from build123d import *

# Parameters (mm, degrees)
F0_W     = 63.5
F0_H     = 82.55
F1_DEPTH = 22.225
F2_R     = 2.38125
F3_DEPTH = 12.7
F4_R     = 2.38125
F5_DEPTH = 63.501
F6_R     = 1.27
F7_DEPTH = 25.4
F8_R     = 3.96875
F9_DEPTH = 3.81


with BuildPart() as f1:
    # F0 (on Front) → F1 (new body, symmetric)
    with BuildSketch(Plane.XZ):
        Rectangle(F0_W, F0_H)
    extrude(amount=F1_DEPTH, both=True)

    # F2 (on face) → F3 (cut)
    with BuildSketch(Plane.XY.offset(41.275)):
        Circle(F2_R)
    extrude(amount=-F3_DEPTH, mode=Mode.SUBTRACT)

    # F4 (on face) → F5 (cut, through all)
    with BuildSketch(Plane(origin=(-31.75, 0, 0), x_dir=(0, -1, 0), z_dir=(-1, 0, 0))):
        with Locations((0, 26.035)):
            Circle(F4_R)
        with Locations((0, -26.035)):
            Circle(F4_R)
    extrude(amount=-F5_DEPTH, mode=Mode.SUBTRACT)

    # F6 (on face) → F7 (cut)
    with BuildSketch(Plane(origin=(0, 22.225, 0), x_dir=(-1, 0, 0), z_dir=(0, 1, 0))):
        with Locations((0, 33.655)):
            Circle(F6_R)
    extrude(amount=-F7_DEPTH, mode=Mode.SUBTRACT)

    # F8 (on face) → F9 (cut)
    with BuildSketch(Plane(origin=(0, 22.225, 0), x_dir=(-1, 0, 0), z_dir=(0, 1, 0))):
        with Locations((0, 33.655)):
            Circle(F8_R)
    extrude(amount=-F9_DEPTH, mode=Mode.SUBTRACT)


solid = f1.part
Design review of the part built by this model. Coordinates are the model's own, in mm. A direction names the side the tool comes from. Give positions to 0.01 mm unless a question says otherwise; leave off trailing zeros. Loops run counter-clockwise (first coordinate to the right, second up) from the corner with the lowest first, then second, coordinate; pieces in that order, holes last. Notation, with made-up numbers: (72.25, 65.5) -> (118.25, 65.5) arc R20 cw to (118.25, 86.5) -> close; hole circle Ø7 at (-30, 81). An arc over 180 degrees is marked (long way). One line per question, with ' | ' between items. Start each with the question number.
(1) For line 1 (Z direction, x = -14, y = 0) (3 decimals); line 2 (Y direction, x = 8.5, z = -26) (3 decimals); line 3 (Z direction, x = 28, y = 2) (3 decimals), list the stretches that pass through material, from the lowest coordinate up.
(2) We need section B-B (x = 0). State the section outline as (y, z) points (1 decimal), and give its area (3 significant figures).
(3) We need section A-A (y = 0). State the section outline as (x, z) points (3 decimals), and give its area (3 significant figures).
(4) For faces 1 (the face through (0, -3.175, 34)), 2 (the face through (1.28, 2.01, 35.01)), 3 (the face through (-0.44, 0.52, -28.36)), list the 3-axis set-ups (+Z, -Z, +X, -X, +Y, -Y) from which the entire face can be reached by the end or side of a thin tool; tool diameter is ignored.
(5) Insertion check: P1, Ø8.5, axis at x = -1.5, z = 35, coming from the +Y side (3 decimals); P2, Ø4, axis at x = 0, z = 33.655, coming from the +Y side (3 decimals). Each pin has a flat end and moves straight along its axis. Give the tip position at first contact, or say it passes through.
(6) Draft analysis for pull direction X (two halves, no side actions). For faces 4 (the face through (31.75, 0, -1)), 5 (the face through (0.275, 10.329, 32.415)), 6 (the face through (0, -22.225, 1)), 7 (the face through (0.94, -2.72, 34.51)), state which applies: +X half, -X half, draft (parallel to the pull), parting line (faces both ways), or undercut.
The answers:
1) line 1: z = -41.275 to -28.416, -23.654 to 23.654, 28.416 to 41.275 | line 2: y = -22.225 to -2.381, 2.381 to 22.225 | line 3: z = -41.275 to -27.327, -24.743 to 24.743, 27.327 to 41.275
2) outline: (-22.2, -41.3) -> (22.2, -41.3) -> (22.2, 29.7) -> (18.4, 29.7) -> (18.4, 32.4) -> (2.4, 32.4) -> (2.4, 28.6) -> (-2.4, 28.6) -> (-2.4, 32.4) -> (-3.2, 32.4) -> (-3.2, 34.9) -> (-2.4, 34.9) -> (-2.4, 41.3) -> (-22.2, 41.3) -> close; (2.4, 34.9) -> (18.4, 34.9) -> (18.4, 37.6) -> (22.2, 37.6) -> (22.2, 41.3) -> (2.4, 41.3) -> close; hole circle Ø4.8 at (0, -26); hole circle Ø4.8 at (0, 26) | area: 3,500 mm^2
3) outline: (-31.75, -41.275) -> (31.75, -41.275) -> (31.75, -28.416) -> (-31.75, -28.416) -> close; (-31.75, -23.654) -> (31.75, -23.654) -> (31.75, 23.654) -> (-31.75, 23.654) -> close; (-31.75, 28.416) -> (31.75, 28.416) -> (31.75, 41.275) -> (2.381, 41.275) -> (2.381, 28.575) -> (-2.381, 28.575) -> (-2.381, 41.275) -> (-31.75, 41.275) -> close | area: 4,580 mm^2
4) face 1: +Y | face 2: +Z | face 3: +X, -X
5) P1: stops at y = 22.225 | P2: stops at y = 18.415
6) face 4: +X half | face 5: undercut | face 6: draft | face 7: undercut
